Here's how the part is built. I have some questions about the finished solid (model axes, mm). A direction names the side the tool comes from. Coordinates: 2 decimals unless noted, no trailing zeros. Write each loop counter-clockwise with the first axis right and the second up, starting at its lowest first coordinate (ties: lowest second). Pieces come first, ordered by that corner, then holes. Notation, with made-up numbers: M 44.5,-5.5 L 85.5,-5.5 A18 ccw 85.5,1.5 Z; hole C 69,14.5 d4. An arc over 180 degrees is marked long. Write each question's results on one line, items separated by ' | '. Start each with the question number.
from build123d import *

# Parameters (mm, degrees)
BOSS_EXTRUDE1_DEPTH = 11
SKETCH2_W           = 8.785422424
SKETCH2_H           = 15.31
BOSS_EXTRUDE2_DEPTH = 11
CUT_EXTRUDE3_REACH  = 74.393
SKETCH3_R           = 1.75
FILLET2_R           = 1.5
FILLET4_R           = 1.5
CUT_EXTRUDE4_REACH  = 48.571
SKETCH5_W           = 4.090875198
SKETCH5_H           = 15.31
FILLET6_R           = 2


with BuildPart() as part:
    # Sketch1 → Boss-Extrude1 (new body)
    with BuildSketch(Plane(origin=(0, 0, 0), x_dir=(1, 0, 0), z_dir=(0, 1, 0))):
        with BuildLine():
            Line((-31.998102942, -0.348436693), (-27.998102942, -0.348436693))
            ThreePointArc((-27.998102942, -0.348436693), (-0.348436693, 27.998102942), (27.998102942, 0.348436693))
            Line((27.998102942, 0.348436693), (31.998102942, 0.348436693))
            ThreePointArc((31.998102942, 0.348436693), (-0.348436693, 31.998102942), (-31.998102942, -0.348436693))
        make_face()
    extrude(amount=BOSS_EXTRUDE1_DEPTH)

    # Sketch2 → Boss-Extrude2 (add, through all)
    with BuildSketch(Plane(origin=(0, 11, 0), x_dir=(1, 0, 0), z_dir=(0, 1, 0))):
        with Locations((27.60539173, 8.003436693)):
            Rectangle(SKETCH2_W, SKETCH2_H)
    extrude(amount=-BOSS_EXTRUDE2_DEPTH)

    # Sketch3 → Cut-Extrude3 (cut, up to next)
    with BuildSketch(Plane(origin=(31.998102942, 0, 0), x_dir=(0, 0, -1), z_dir=(1, 0, 0)), mode=Mode.PRIVATE) as cut_extrude3_sk1:
        with Locations((3.439433815, 5.5)):
            Circle(SKETCH3_R)
    cut_extrude3_tool1 = extrude(cut_extrude3_sk1.sketch, amount=-CUT_EXTRUDE3_REACH, mode=Mode.PRIVATE) & part.part
    # Sketch3 → Cut-Extrude3 (cut, up to next)
    with BuildSketch(Plane(origin=(31.998102942, 0, 0), x_dir=(0, 0, -1), z_dir=(1, 0, 0)), mode=Mode.PRIVATE) as cut_extrude3_sk2:
        with Locations((12.439433815, 5.5)):
            Circle(SKETCH3_R)
    cut_extrude3_tool2 = extrude(cut_extrude3_sk2.sketch, amount=-CUT_EXTRUDE3_REACH, mode=Mode.PRIVATE) & part.part
    add(cut_extrude3_tool1.solids().sort_by_distance((31.998103, 5.5, -3.439434))[0], mode=Mode.SUBTRACT)
    add(cut_extrude3_tool2.solids().sort_by_distance((31.998103, 5.5, -12.439434))[0], mode=Mode.SUBTRACT)

    # Fillet2
    fillet2_edges = [part.edges().sort_by_distance(p)[0] for p in [
        (23.212680518, 5.5, -15.658436693),
    ]]
    fillet(fillet2_edges, radius=FILLET2_R)

    # Fillet4
    fillet4_edges = [part.edges().sort_by_distance(p)[0] for p in [
        (-31.998102942, 5.5, 0.348436693),
        (-27.998102942, 5.5, 0.348436693),
    ]]
    fillet(fillet4_edges, radius=FILLET4_R)

    # Sketch5 → Cut-Extrude4 (cut, up to next)
    with BuildSketch(Plane(origin=(0, 11, 0), x_dir=(1, 0, 0), z_dir=(0, 1, 0)), mode=Mode.PRIVATE) as cut_extrude4_sk1:
        with Locations((29.952665343, 8.003436693)):
            Rectangle(SKETCH5_W, SKETCH5_H)
    cut_extrude4_tool1 = extrude(cut_extrude4_sk1.sketch, amount=-CUT_EXTRUDE4_REACH, mode=Mode.PRIVATE) & part.part
    add(cut_extrude4_tool1.solids().sort_by_distance((29.952665, 11, -8.003437))[0], mode=Mode.SUBTRACT)

    # Fillet6
    fillet6_edges = [part.edges().sort_by_distance(p)[0] for p in [
        (27.907227744, 5.5, -15.658436693),
    ]]
    fillet(fillet6_edges, radius=FILLET6_R)


solid = part.part
1) I want a section at D-D, the plane z = -3.5. Write out the boundary of the cut face in (x, y), then the cut area to 3 significant figures.
2) For pin 1 Ø12 at (x, z) = (20.5, -4) entering from -Y; pin 2 Ø5 at (x, y) = (-3, 9.5) entering from +Z; pin 3 Ø3 at (y, z) = (5.5, -12.44) entering from +X; pin 4 Ø5.5 at (y, z) = (4.5, -8) entering from -X, each with a flat end and sliding along its axis, tell me the tip position at first contact or that it passes through.
3) I want a section at C-C, the plane y = 2.75. Write out the boundary of the cut face in (x, z).
4) For faces 1 (the cylindrical face through (25.59, 3.95, -13.25)), 2 (the flat face through (27.907, 6, -8)), 3 (the flat face through (23.213, 6, -8)), which set-ups out of +Z, -Z, +X, -X, +Y, -Y let a thin tool reach every point of the face, with its end or its side?
5) I want a section at B-B, the plane z = -18.5. Write out the boundary of the cut face in (x, y), then the cut area to 3 significant figures.
6) I want a section at A-A, the plane y = 5.5. Write out the boundary of the cut face in (x, z).
7) Please list where these lines run through material, in increasing order: line 1 (X direction, y = 0.5, z = -16); line 2 (X direction, y = 2.5, z = -10); line 3 (X direction, y = 6.75, z = -3.5). Write a range as [from, to].
8) We'd pull the mould along Y, two halves only. Please class faces 4 (the cylindrical face through (25.59, 3.79, -3.06)), 5 (the flat face through (-2, 0, -29)), 6 (the flat face through (26, 6, -0.348)): pulls with the +Y half, pulls with the -Y half, needs draft (parallel to the pull), parting line crosses it, or undercut.
Output:
1) outline: M -31.81,0 L -27.78,0 L -27.78,11 L -31.81,11 Z; M 23.21,0 L 27.91,0 L 27.91,3.75 L 23.21,3.75 Z; M 23.21,7.25 L 27.91,7.25 L 27.91,11 L 23.21,11 Z | area: 79.5 mm2
2) pin 1: stops at y = 0 | pin 2: stops at z = -27.45 | pin 3: stops at x = -24.28 | pin 4: stops at x = -31.57
3) outline: M -31.98,-1.21 A32 ccw 27.63,-16.14 A2 ccw 27.91,-15.13 L 27.91,-0.35 L 23.21,-0.35 L 23.21,-15.19 A1.5 cw 22.94,-16.05 A28 cw -27.98,-1.09 A1.5 ccw -29.48,0.35 L -30.48,0.35 A1.5 ccw Z
4) face 1: +X | face 2: +Z, -Z, +X, +Y, -Y | face 3: +Z, +Y, -Y
5) outline: M -26.11,0 L -21.02,0 L -21.02,11 L -26.11,11 Z; M 21.02,0 L 26.11,0 L 26.11,11 L 21.02,11 Z | area: 112 mm2
6) outline: M -31.98,-1.21 A32 ccw 27.63,-16.14 A2 ccw 27.91,-15.13 L 27.91,-14.19 L 23.21,-14.19 L 23.21,-15.19 A1.5 cw 22.94,-16.05 A28 cw -27.98,-1.09 A1.5 ccw -29.48,0.35 L -30.48,0.35 A1.5 ccw Z; M 23.21,-10.69 L 27.91,-10.69 L 27.91,-5.19 L 23.21,-5.19 Z; M 23.21,-1.69 L 27.91,-1.69 L 27.91,-0.35 L 23.21,-0.35 Z
7) line 1: x = [-27.71, -22.98], [22.98, 27.71] | line 2: x = [-30.4, -26.15], [23.21, 27.91] | line 3: x = [-31.81, -27.78]
8) face 4: undercut | face 5: pulls with the -Y half | face 6: needs draft
